```python
from build123d import *

# Parameters (mm, degrees)
PAD002_DEPTH  = 5
SKETCH008_R   = 11
HOLE001_DEPTH = 5
SKETCH009_R   = 1.4
HOLE002_DEPTH = 5
SKETCH010_R   = 3.25
HOLE003_DEPTH = 1.7


with BuildPart() as part:
    # Sketch007 → Pad002 (new body)
    with BuildSketch(Plane.XY):
        with BuildLine():
            Line((-176, -1), (176, -1))
            ThreePointArc((179, -4), (178.12132, -1.87868), (176, -1))
            Line((179, -4), (179, -225))
            ThreePointArc((176, -228), (178.12132, -227.12132), (179, -225))
            Line((176, -228), (-176, -228))
            ThreePointArc((-179, -225), (-178.12132, -227.12132), (-176, -228))
            Line((-179, -225), (-179, -4))
            ThreePointArc((-176, -1), (-178.12132, -1.87868), (-179, -4))
        make_face()
    extrude(amount=PAD002_DEPTH)

    # Sketch008 → Hole001 (cut)
    with BuildSketch(Plane.XY):
        with Locations((-142.75, -17.7)):
            Circle(SKETCH008_R)
        with Locations((-120.25, -17.7)):
            Circle(SKETCH008_R)
        with Locations((-69.5, -37.5)):
            Circle(SKETCH008_R)
        with Locations((-69.5, -67.5)):
            Circle(SKETCH008_R)
        with Locations((-100, -77.5)):
            Circle(SKETCH008_R)
        with Locations((-125, -102.5)):
            Circle(SKETCH008_R)
        with Locations((-39.5, -77.5)):
            Circle(SKETCH008_R)
        with Locations((5, -80)):
            Circle(SKETCH008_R)
        with Locations((35, -70)):
            Circle(SKETCH008_R)
        with Locations((65, -65)):
            Circle(SKETCH008_R)
        with Locations((95, -70)):
            Circle(SKETCH008_R)
        with Locations((125, -75)):
            Circle(SKETCH008_R)
        with Locations((-10, -137.5)):
            Circle(SKETCH008_R)
        with Locations((20, -127.5)):
            Circle(SKETCH008_R)
        with Locations((35, -102.5)):
            Circle(SKETCH008_R)
        with Locations((65, -97.5)):
            Circle(SKETCH008_R)
        with Locations((95, -102.5)):
            Circle(SKETCH008_R)
        with Locations((125, -107.5)):
            Circle(SKETCH008_R)
    extrude(amount=HOLE001_DEPTH, mode=Mode.SUBTRACT)

    # Sketch009 → Hole002 (cut)
    with BuildSketch(Plane.XY):
        with Locations((0, -210)):
            Circle(SKETCH009_R)
        with Locations((160, -210)):
            Circle(SKETCH009_R)
        with Locations((160, -10)):
            Circle(SKETCH009_R)
        with Locations((-160, -210)):
            Circle(SKETCH009_R)
        with Locations((-160, -10)):
            Circle(SKETCH009_R)
        with Locations((0, -110)):
            Circle(SKETCH009_R)
    extrude(amount=HOLE002_DEPTH, mode=Mode.SUBTRACT)

    # Sketch010 → Hole003 (cut)
    with BuildSketch(Plane(origin=(0, 0, 5), x_dir=(-1, 0, 0), z_dir=(0, 0, 1))):
        with Locations((0, 110)):
            Circle(SKETCH010_R)
    extrude(amount=-HOLE003_DEPTH, mode=Mode.SUBTRACT)


with BuildPart() as part_1:
    # Body001 placement: moved
    add(part.part.moved(Location((0, 0, 13.01))))


solid = part_1.part
```
Design review of the part built by this model. Coordinates are the model's own, in mm. A direction names the side the tool comes from. Round coordinates to 2 decimals unless told otherwise and drop trailing zeros. Order: outer loops, then holes, each group sorted by start corner. A loop starts at its lowest first (then second) coordinate and runs counter-clockwise, first axis right, second up. Notation, with made-up numbers: (8.25, -40) - (52.25, -40) arc R11 ccw to (52.25, -23) - close; hole circle Ø6 at (13, 50.5). An arc over 180 degrees is marked (long way). Return JSON: item names as keys, results as strings.
Q1. Machinability: for faces 1 (the cylindrical face through (-80.49, -37.02, 15.48)), 2 (the flat face through (-0.7, -108.6, 16.31)), which of the approach directions +Z, -Z, +X, -X, +Y, -Y give a long, thin tool a straight path to every point of the face, cutting with its end or side? Answer none if there is none.
Computed values:
{"face 1": "+Z, -Z", "face 2": "+Z"}
Q2. Consider section C-C on x = -120.25. Write out the cut boundary in (y, z), plus the area to 3 significant figures.
Computed values:
{"outline": "(-228, 13.01) - (-112.42, 13.01) - (-112.42, 18.01) - (-228, 18.01) - close; (-92.58, 13.01) - (-28.7, 13.01) - (-28.7, 18.01) - (-92.58, 18.01) - close; (-6.7, 13.01) - (-1, 13.01) - (-1, 18.01) - (-6.7, 18.01) - close", "area": "926 mm2"}
Q3. Consider section B-B on y = -42. Write out the cut boundary in (x, z), plus the area to 3 significant figures.
Computed values:
{"outline": "(-179, 13.01) - (-79.54, 13.01) - (-79.54, 18.01) - (-179, 18.01) - close; (-59.46, 13.01) - (179, 13.01) - (179, 18.01) - (-59.46, 18.01) - close", "area": "1,690 mm2"}
Q4. Wall thickness on L1, parallel to Y at x = 35, z = 14.2; L2, parallel to Y at x = -70, z = 17.05; L3, parallel to X at y = -85, z = 17.45: over which ranges is each line inside the solid? List them lowest first. Write a range as [from, to].
Computed values:
{"L1": "y = [-228, -113.5], [-91.5, -81], [-59, -1]", "L2": "y = [-228, -78.49], [-56.51, -48.49], [-26.51, -1]", "L3": "x = [-179, -108.05], [-91.95, -47.55], [-31.45, -4.8], [14.8, 120.42], [129.58, 179]"}
Q5. Consider section D-D on x = 41. Write out the cut boundary in (y, z), plus the area to 3 significant figures.
Computed values:
{"outline": "(-228, 13.01) - (-111.72, 13.01) - (-111.72, 18.01) - (-228, 18.01) - close; (-93.28, 13.01) - (-79.22, 13.01) - (-79.22, 18.01) - (-93.28, 18.01) - close; (-60.78, 13.01) - (-1, 13.01) - (-1, 18.01) - (-60.78, 18.01) - close", "area": "951 mm2"}
Q6. For pin 1 Ø3 at (x, y) = (0.5, -111) entering from +Z; pin 2 Ø3.5 at (x, y) = (-160, -210) entering from -Z, all flat-tipped, find the tip position at first contact; note any pin that passes through.
Computed values:
{"pin 1": "stops at z = 16.31", "pin 2": "stops at z = 13.01"}
Q7. The part is to be moulded in two halves that separate along Y. For faces 3 (the flat face through (3, -113, 18.01)), 4 (the cylindrical face through (114, -75, 15)), say which applies: pulls with the +Y half, pulls with the -Y half, needs draft (parallel to the pull), parting line crosses it, or undercut.
Computed values:
{"face 3": "needs draft", "face 4": "undercut"}
Q8. Consider section A-A on z = 15.05. Give the number of separate pieces and of enclosed holes in the cut face, plus the area to 3 significant figures.
Computed values:
{"separate pieces": "1", "enclosed holes": "24", "area": "74,400 mm2"}
